The model under review builds one solid part; all positions refer to its coordinate system, in mm. A direction names the side the tool comes from. Give positions to 0.01 mm unless a question says otherwise; leave off trailing zeros. Order: outer loops, then holes, each group sorted by start corner. A loop starts at its lowest first (then second) coordinate and runs counter-clockwise, first axis right, second up. Notation, with made-up numbers: (44.5, -4) - (78.5, -4) arc R23 ccw to (78.5, 25) - close; hole circle Ø11 at (-14, 37.5). An arc over 180 degrees is marked (long way). Answer as CSV lines item,"result". Start each with the question number.
from build123d import *

# Parameters (mm, degrees)
BOSS_EXTRUDE1_DEPTH  = 30.2
CUT_EXTRUDE3_DEPTH   = 6.9
SKETCH10_R           = 7.5
BOSS_EXTRUDE6_DEPTH  = 4.1
SKETCH11_R           = 4
BOSS_EXTRUDE7_DEPTH  = 6.9
BOSS_EXTRUDE8_DEPTH  = 8.9
BOSS_EXTRUDE9_DEPTH  = 2
BOSS_EXTRUDE10_DEPTH = 1.8
CUT_EXTRUDE5_DEPTH   = 4
SKETCH23_R           = 1.75
CUT_EXTRUDE6_DEPTH   = 7


with BuildPart() as part:
    # Sketch1 → Boss-Extrude1 (new body)
    with BuildSketch(Plane(origin=(0, 0, 0), x_dir=(0, 0, -1), z_dir=(1, 0, 0))):
        Polygon((0, 0), (66.1, 0), (66.1, 42.1), (74.4, 42.1), (74.4, 46), (66.1, 46), (66.1, 59.3), (12.213560369, 59.3), (12.213560369, 52.65), (0, 52.65), (0, 46), (-8.3, 46), (-8.3, 42.1), (0, 42.1), align=None)
    extrude(amount=BOSS_EXTRUDE1_DEPTH)

    # Sketch9 → Cut-Extrude3 (cut)
    with BuildSketch(Plane(origin=(0, 46, 0), x_dir=(1, 0, 0), z_dir=(0, 1, 0))):
        with BuildLine():
            Line((22, 74.4), (22, 72.137458609))
            ThreePointArc((22, 72.137458609), (24, 67.5), (26, 72.137458609))
            Line((26, 72.137458609), (26, 74.4))
            Line((26, 74.4), (24, 74.4))
            Line((24, 74.4), (22, 74.4))
        make_face()
        with BuildLine():
            Line((6.2, 74.4), (4.2, 74.4))
            Line((4.2, 74.4), (4.2, 72.137458609))
            ThreePointArc((4.2, 72.137458609), (6.2, 67.5), (8.2, 72.137458609))
            Line((8.2, 72.137458609), (8.2, 74.4))
            Line((8.2, 74.4), (6.2, 74.4))
        make_face()
        with BuildLine():
            Line((24, -8.3), (26, -8.3))
            Line((26, -8.3), (26, -6.037458609))
            ThreePointArc((26, -6.037458609), (24, -1.4), (22, -6.037458609))
            Line((22, -6.037458609), (22, -8.3))
            Line((22, -8.3), (24, -8.3))
        make_face()
        with BuildLine():
            Line((8.2, -8.3), (8.2, -6.037458609))
            ThreePointArc((8.2, -6.037458609), (6.2, -1.4), (4.2, -6.037458609))
            Line((4.2, -6.037458609), (4.2, -8.3))
            Line((4.2, -8.3), (6.2, -8.3))
            Line((6.2, -8.3), (8.2, -8.3))
        make_face()
    extrude(amount=-CUT_EXTRUDE3_DEPTH, mode=Mode.SUBTRACT)

    # Sketch10 → Boss-Extrude6 (add)
    with BuildSketch(Plane(origin=(0, 59.3, 0), x_dir=(1, 0, 0), z_dir=(0, 1, 0))):
        with Locations((15.1, 50.25)):
            Circle(SKETCH10_R)
    extrude(amount=BOSS_EXTRUDE6_DEPTH)

    # Sketch11 → Boss-Extrude7 (add)
    with BuildSketch(Plane(origin=(0, 63.4, 0), x_dir=(1, 0, 0), z_dir=(0, 1, 0))):
        with Locations((15.1, 50.25)):
            Circle(SKETCH11_R)
    extrude(amount=BOSS_EXTRUDE7_DEPTH)

    # Sketch14 → Boss-Extrude8 (add)
    with BuildSketch(Plane(origin=(0, 61.3, 0), x_dir=(1, 0, 0), z_dir=(0, 1, 0))):
        with BuildLine():
            Line((0, 39.156780185), (15.1, 39.156780185))
            Line((15.1, 39.156780185), (19.1, 39.156780185))
            Line((19.1, 39.156780185), (19.1, 15.178872415))
            ThreePointArc((19.1, 15.178872415), (15.1, 11.178872415), (11.1, 15.178872415))
            Line((11.1, 15.178872415), (0, 15.178872415))
            Line((0, 15.178872415), (0, 39.156780185))
        make_face()
    extrude(amount=-BOSS_EXTRUDE8_DEPTH)

    # Sketch17 → Boss-Extrude9 (add)
    with BuildSketch(Plane(origin=(0, 59.3, 0), x_dir=(1, 0, 0), z_dir=(0, 1, 0))):
        Polygon((0, 12.213560369), (15.153721143, 12.213560369), (15.1, 15.178872415), (0, 15.178872415), align=None)
    extrude(amount=BOSS_EXTRUDE9_DEPTH)

    # Sketch18 → Boss-Extrude10 (add)
    with BuildSketch(Plane(origin=(0, 46, 0), x_dir=(1, 0, 0), z_dir=(0, 1, 0))):
        Polygon((15.1, 74.4), (16.6, 74.4), (16.6, 66.1), (13.6, 66.1), (13.6, 74.4), align=None)
        Polygon((13.6, -8.3), (15.1, -8.3), (16.6, -8.3), (16.6, 0), (13.6, 0), align=None)
    extrude(amount=BOSS_EXTRUDE10_DEPTH)

    # Sketch22 → Cut-Extrude5 (cut)
    with BuildSketch(Plane(origin=(16.6, 0, 0), x_dir=(0, 0, -1), z_dir=(1, 0, 0))):
        Polygon((74.4, 46), (72.6, 47.8), (74.4, 47.8), align=None)
        Polygon((-8.3, 47.8), (-8.3, 46), (-6.5, 47.8), align=None)
    extrude(amount=-CUT_EXTRUDE5_DEPTH, mode=Mode.SUBTRACT)

    # Sketch23 → Cut-Extrude6 (cut)
    with BuildSketch(Plane(origin=(0, 70.3, 0), x_dir=(1, 0, 0), z_dir=(0, 1, 0))):
        with Locations((15.1, 50.25)):
            Circle(SKETCH23_R)
    extrude(amount=-CUT_EXTRUDE6_DEPTH, mode=Mode.SUBTRACT)


solid = part.part
Item 1: Clearance check with flat-ended pins moving along their axes: pin 1 (4 mm diameter, centred on x = 4.5, z = -70.5, fed in from +Y); pin 2 (4.5 mm diameter, centred on x = 7.5, y = 58, fed in from +Z); pin 3 (7.5 mm diameter, centred on x = 25, y = 54.5, fed in from +Z); pin 4 (2.5 mm diameter, centred on x = 23.5, z = -70, fed in from +Y). State where each tip first meets the part, or that it passes through.
Item 2: Take a section at A-A on z = 4.15. Write out the cut boundary in (x, y), and give its area (3 significant figures).
Item 3: For line 1 along X through (y, z) = (43.25, 4.15); line 2 along Z through (x, y) = (22, 55); line 3 along Z through (x, y) = (24.5, 31.5), list the stretches that pass through material, from the lowest coordinate up.
Item 4: Take a section at B-B on y = 44.5. Write out the cut boundary in (x, z).
Item 5: Take a section at D-D on y = 65.5. Write out the cut boundary in (x, z).
Item 6: Machinability: for faces 1 (the face through (6, 57, -12.214)), 2 (the face through (9, 61.3, -25)), 3 (the face through (15, 21, -66.1)), which of the approach directions +Z, -Z, +X, -X, +Y, -Y give a long, thin tool a straight path to every point of the face, cutting with its end or side? Answer none if there is none.
Item 7: Mouldability with a two-part tool opening along X and no side actions: class faces 4 (the face through (8.2, 44, 7)), 5 (the face through (22, 46, 2)), 6 (the face through (13.6, 47, 4)) as released by +X, released by -X, zero draft, split by the parting line, or undercut.
Data:
1,pin 1,"stops at y = 46"
1,pin 2,"stops at z = -12.21"
1,pin 3,"stops at z = 0"
1,pin 4,"passes through"
2,outline,"(0, 42.1) - (3.45, 42.1) - (3.45, 46) - (0, 46) - close; (8.95, 42.1) - (21.25, 42.1) - (21.25, 46) - (16.6, 46) - (16.6, 47.8) - (13.6, 47.8) - (13.6, 46) - (8.95, 46) - close; (26.75, 42.1) - (30.2, 42.1) - (30.2, 46) - (26.75, 46) - close"
2,area,"80.3 mm^2"
3,line 1,"x = 0 to 3.45, 8.95 to 21.25, 26.75 to 30.2"
3,line 2,"z = -66.1 to -12.21"
3,line 3,"z = -66.1 to 0"
4,outline,"(0, -74.4) - (4.2, -74.4) - (4.2, -72.14) arc R2.75 cw (long way) to (8.2, -72.14) - (8.2, -74.4) - (22, -74.4) - (22, -72.14) arc R2.75 cw (long way) to (26, -72.14) - (26, -74.4) - (30.2, -74.4) - (30.2, 8.3) - (26, 8.3) - (26, 6.04) arc R2.75 cw (long way) to (22, 6.04) - (22, 8.3) - (8.2, 8.3) - (8.2, 6.04) arc R2.75 cw (long way) to (4.2, 6.04) - (4.2, 8.3) - (0, 8.3) - close"
5,outline,"circle Ø8 at (15.1, -50.25); hole circle Ø3.5 at (15.1, -50.25)"
6,face 1,"+Z, -X, +Y"
6,face 2,"+Z, +X, -X, +Y"
6,face 3,"-Z, +X, -X, -Y"
7,face 4,"undercut"
7,face 5,"zero draft"
7,face 6,"released by -X"
